Job drawing, mm, ordinate dimensions from the low corner. One solid piece. Give positions to 0.01 mm unless a question says otherwise; leave off trailing zeros. Order: outer loops, then holes, each group sorted by start corner. A loop starts at its lowest first (then second) coordinate and runs counter-clockwise, first axis right, second up. Notation, with made-up numbers: M 77,19 L 112,19 A11 ccw 112,34 Z; hole C 57.5,9.5 d8. An arc over 180 degrees is marked long. Put each result on its own line as item: value. Start each with the question number.
1) Cut at D-D (z = 34.5). Write the cut outline in (x, y).
2) Cut at C-C (x = 41). Write the cut outline in (y, z).
3) Cut at B-B (y = 0.75). Write the cut outline in (x, z), and give its area (3 significant figures).
4) Drill centre lines: line 1 (X direction, y = 0.8, z = 3); line 2 (Z direction, x = 28, y = 1.55); line 3 (X direction, y = 0.85, z = 36). Where is each one in solid material? Low to high. Write a range as [from, to].
5) Cut at A-A (z = 4). Write the cut outline in (x, y), and give its area (3 significant figures).
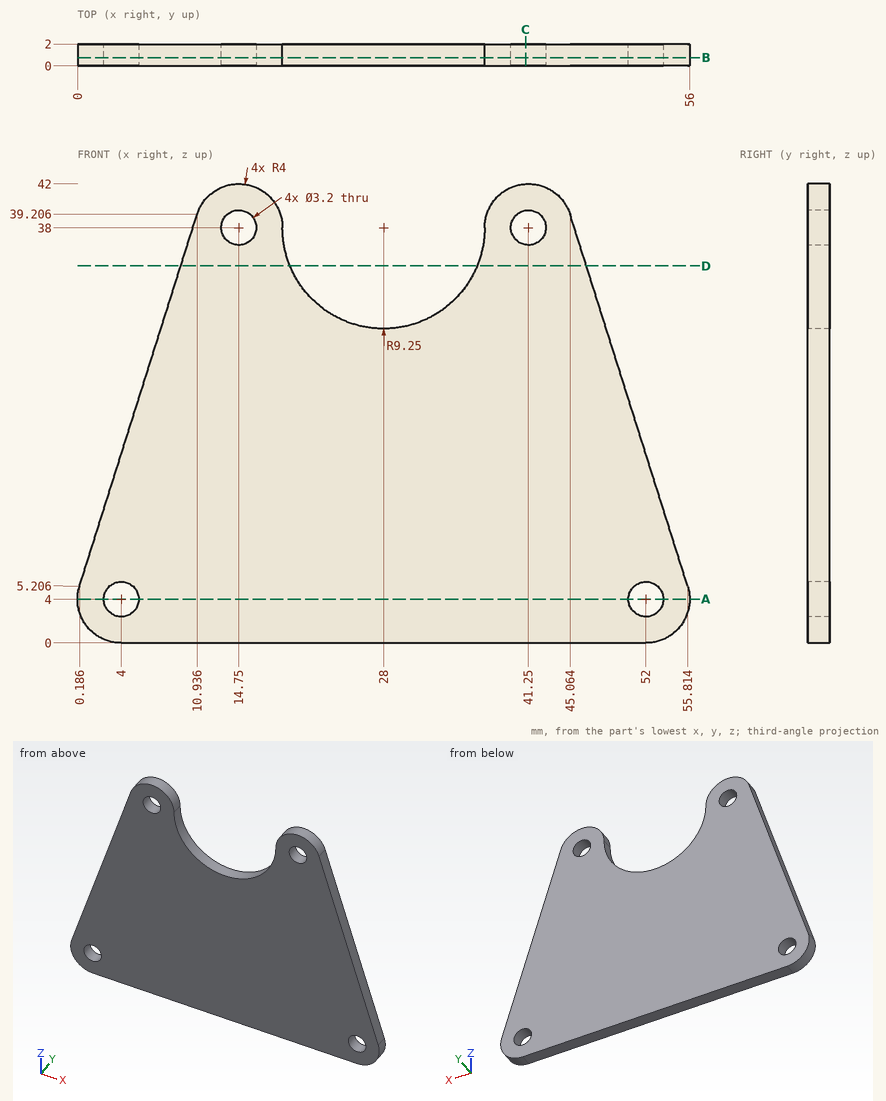
Solution:
1. outline: M 9.45,0 L 19.44,0 L 19.44,2 L 9.45,2 Z; M 36.56,0 L 46.55,0 L 46.55,2 L 36.56,2 Z
2. outline: M 0,0 L 2,0 L 2,36.42 L 0,36.42 Z; M 0,39.58 L 2,39.58 L 2,41.99 L 0,41.99 Z
3. outline: M 0.19,5.21 A4 ccw 4,0 L 52,0 A4 ccw 55.81,5.21 L 45.06,39.21 A4 ccw 37.25,38 A9.25 cw 18.75,38 A4 ccw 10.94,39.21 Z; hole C 4,4 d3.2; hole C 14.75,38 d3.2; hole C 41.25,38 d3.2; hole C 52,4 d3.2
3. area: 1,650 mm²
4. line 1: [0.13, 2.75], [5.25, 50.75], [53.25, 55.87]
4. line 2: [0, 28.75]
4. line 3: [9.92, 18.97], [37.03, 46.08]
5. outline: M 0,0 L 2.4,0 L 2.4,2 L 0,2 Z; M 5.6,0 L 50.4,0 L 50.4,2 L 5.6,2 Z; M 53.6,0 L 56,0 L 56,2 L 53.6,2 Z
5. area: 99.2 mm²
